```python
from build123d import *

# Parameters (mm, degrees)
SKETCH1_R                    = 1.6
BASE_DEPTH                   = 6
PTFE_CLAMP_3MM_OD_DEPTH      = 32.5
PTFE_CLAMP_1_6MM_OD_DEPTH    = 32.500000138
SKETCH3_R                    = 2.9
RUTHEX_M3_INSERT_HOLE_DEPTH  = 8.3
SIDE_PROFILE_DEPTH           = 4.4
ANGLE_CONSTRAINT_BACK_START  = -4
ANGLE_CONSTRAINT_BACK_DEPTH  = 8.4
ANGLE_CONSTRAINT_FRONT_START = -4
ANGLE_CONSTRAINT_FRONT_DEPTH = 8.4
FILLET4_R                    = 1
FILLET5_R                    = 2
FILLET4_OF_MIRROR4_R         = 1
FILLET5_OF_MIRROR4_R         = 2


with BuildPart() as part:
    # Sketch1 → base (new, symmetric)
    with BuildSketch(Plane(origin=(0, 0, 0), x_dir=(0, 0, -1), z_dir=(1, 0, 0))):
        with BuildLine():
            Line((7.5, 0), (-7.5, 0))
            Line((-7.5, 0), (-7.5, 22.5))
            ThreePointArc((-7.5, 22.5), (0, 30), (7.5, 22.5))
            Line((7.5, 22.5), (7.5, 0))
        make_face()
        with Locations((0, 22.5)):
            Circle(SKETCH1_R, mode=Mode.SUBTRACT)
    extrude(amount=BASE_DEPTH, both=True)

    # Sketch2 → PTFE_clamp_3mm_OD (cut, through all)
    with BuildSketch(Plane.XZ):
        with BuildLine():
            Line((0, -7.5), (1.202081528, -7.5))
            ThreePointArc((1.202081528, -7.5), (1.570595205, -5.647356637), (0, -4.597918472))
            Line((0, -4.597918472), (0, -7.5))
        make_face()
        with BuildLine():
            Line((-1.202081528, -7.5), (0, -7.5))
            Line((0, -7.5), (0, -4.597918472))
            ThreePointArc((0, -4.597918472), (-1.570595205, -5.647356637), (-1.202081528, -7.5))
        make_face()
        with BuildLine():
            Line((0, -7.5), (1.202081528, -7.5))
            ThreePointArc((1.202081528, -7.5), (1.570595205, -5.647356637), (0, -4.597918472))
            Line((0, -4.597918472), (0, -7.5))
        make_face()
        with BuildLine():
            Line((-1.202081528, -7.5), (0, -7.5))
            Line((0, -7.5), (0, -4.597918472))
            ThreePointArc((0, -4.597918472), (-1.570595205, -5.647356637), (-1.202081528, -7.5))
        make_face()
    extrude(amount=-PTFE_CLAMP_3MM_OD_DEPTH, mode=Mode.SUBTRACT)

    # Sketch2<3> → PTFE_clamp_1.6mm_OD (cut, through all)
    with BuildSketch(Plane.XZ):
        with BuildLine():
            ThreePointArc((-0.707106781, 7.5), (-0.923879533, 6.410209786), (0, 5.792893219))
            Line((0, 5.792893219), (0, 7.5))
            Line((0, 7.5), (-0.707106781, 7.5))
        make_face()
        with BuildLine():
            Line((0, 7.5), (0, 5.792893219))
            ThreePointArc((0, 5.792893219), (0.923879533, 6.410209786), (0.707106781, 7.5))
            Line((0.707106781, 7.5), (0, 7.5))
        make_face()
        with BuildLine():
            ThreePointArc((-0.707106781, 7.5), (-0.923879533, 6.410209786), (0, 5.792893219))
            Line((0, 5.792893219), (0, 7.5))
            Line((0, 7.5), (-0.707106781, 7.5))
        make_face()
        with BuildLine():
            Line((0, 7.5), (0, 5.792893219))
            ThreePointArc((0, 5.792893219), (0.923879533, 6.410209786), (0.707106781, 7.5))
            Line((0.707106781, 7.5), (0, 7.5))
        make_face()
    extrude(amount=-PTFE_CLAMP_1_6MM_OD_DEPTH, mode=Mode.SUBTRACT)

    # Sketch3 → ruthex_m3_insert_hole (cut)
    with BuildSketch(Plane.XZ):
        with Locations(Location((0, 0, 0), (0, 0, 270))):
            Circle(SKETCH3_R)
    extrude(amount=-RUTHEX_M3_INSERT_HOLE_DEPTH, mode=Mode.SUBTRACT)

    # Sketch4 → side_profile (add)
    with BuildSketch(Plane.ZY.offset(6)):
        Polygon((-8, 0), (7.5, 0), (7.5, 19.490381057), (3.077350269, 11.830127019), (-2.5, 11.830127019), (-8, 17.330127019), align=None)
    side_profile = extrude(amount=SIDE_PROFILE_DEPTH)

    # Sketch4<4> → angle_constraint_back (add)
    with BuildSketch(Plane.ZY.offset(6).offset(ANGLE_CONSTRAINT_BACK_START)):
        Polygon((-10.5, 0), (-8, 0), (-8, 17.330127019), (-8, 26.5), (-10.5, 26.5), align=None)
    angle_constraint_back = extrude(amount=ANGLE_CONSTRAINT_BACK_DEPTH)

    # Sketch4<6> → angle_constraint_front (add)
    with BuildSketch(Plane.ZY.offset(6).offset(ANGLE_CONSTRAINT_FRONT_START)):
        Polygon((7.5, 19.490381057), (7.5, 0), (10.5, 0), (10.5, 24.686533479), align=None)
    angle_constraint_front = extrude(amount=ANGLE_CONSTRAINT_FRONT_DEPTH)

    # Fillet4
    fillet4_edges = [part.edges().sort_by_distance(p)[0] for p in [
        (-6.2, 26.5, -8),
        (-6.2, 0, -10.5),
        (-6.2, 26.5, -10.5),
        (-6.2, 24.686533479, 10.5),
        (-6.2, 0, 10.5),
    ]]
    fillet(fillet4_edges, radius=FILLET4_R)

    # Fillet5
    # the kernel refuses this fillet: 2 mm, written as the material it adds along each edge
    with BuildSketch(Plane(origin=(-3.113248654, 11.830127019, 3.077350269), x_dir=(0, 0.8660254037844377, 0.5000000000000013), z_dir=(-1, 0, 0))) as fillet5_piece_1:
        with BuildLine():
            CenterArc((FILLET5_R * 0.57735026919, FILLET5_R), FILLET5_R, 210, 60)
            Line((-FILLET5_R * 0.288675134595, FILLET5_R * 0.5), (0, 0))
            Line((0, 0), (FILLET5_R * 0.57735026919, 0))
        make_face()
    extrude(amount=7.286751346)
    with BuildSketch(Plane(origin=(-3.928932188, 11.830127019, -2.5), x_dir=(0, 0.7071067811865489, -0.7071067811865462), z_dir=(-1, 0, 0))) as fillet5_piece_2:
        with BuildLine():
            CenterArc((FILLET5_R * 0.414213562373, -FILLET5_R), FILLET5_R, 90, 45)
            Line((-FILLET5_R * 0.292893218813, -FILLET5_R * 0.292893218813), (0, 0))
            Line((0, 0), (FILLET5_R * 0.414213562373, 0))
        make_face()
    extrude(amount=6.471067812)
    with BuildSketch(Plane(origin=(-6, 17.330127019, -8), x_dir=(0, 1, 0), z_dir=(-1, 0, 0))) as fillet5_piece_3:
        with BuildLine():
            CenterArc((FILLET5_R * 0.414213562373, -FILLET5_R), FILLET5_R, 90, 45)
            Line((-FILLET5_R * 0.292893218813, -FILLET5_R * 0.292893218813), (0, 0))
            Line((0, 0), (FILLET5_R * 0.414213562373, 0))
        make_face()
    extrude(amount=4.4)

    # Mirror4: side_profile, angle_constraint_back, angle_constraint_front across plane
    add(side_profile.mirror(Plane(origin=(0, 0, 0), x_dir=(0, 0, 1), z_dir=(1, 0, 0))))
    add(angle_constraint_back.mirror(Plane(origin=(0, 0, 0), x_dir=(0, 0, 1), z_dir=(1, 0, 0))))
    add(angle_constraint_front.mirror(Plane(origin=(0, 0, 0), x_dir=(0, 0, 1), z_dir=(1, 0, 0))))

    # Fillet4 of Mirror4
    fillet4_of_mirror4_edges = [part.edges().sort_by_distance(p)[0] for p in [
        (6.2, 26.5, -8),
        (6.2, 0, -10.5),
        (6.2, 26.5, -10.5),
        (6.2, 24.686533479, 10.5),
        (6.2, 0, 10.5),
    ]]
    fillet(fillet4_of_mirror4_edges, radius=FILLET4_OF_MIRROR4_R)

    # Fillet5 of Mirror4
    # the kernel refuses this fillet: 2 mm, written as the material it adds along each edge
    with BuildSketch(Plane(origin=(3.113248654, 11.830127019, 3.077350269), x_dir=(0, 0.8660254037844386, 0.5000000000000002), z_dir=(1, 0, 0))) as fillet5_of_mirror4_piece_1:
        with BuildLine():
            CenterArc((FILLET5_OF_MIRROR4_R * 0.57735026919, -FILLET5_OF_MIRROR4_R), FILLET5_OF_MIRROR4_R, 90, 60)
            Line((-FILLET5_OF_MIRROR4_R * 0.288675134595, -FILLET5_OF_MIRROR4_R * 0.5), (0, 0))
            Line((0, 0), (FILLET5_OF_MIRROR4_R * 0.57735026919, 0))
        make_face()
    extrude(amount=7.286751346)
    with BuildSketch(Plane(origin=(3.928932188, 11.830127019, -2.5), x_dir=(0, 0, 1), z_dir=(1, 0, 0))) as fillet5_of_mirror4_piece_2:
        with BuildLine():
            CenterArc((FILLET5_OF_MIRROR4_R * 0.414213562373, -FILLET5_OF_MIRROR4_R), FILLET5_OF_MIRROR4_R, 90, 45)
            Line((-FILLET5_OF_MIRROR4_R * 0.292893218813, -FILLET5_OF_MIRROR4_R * 0.292893218813), (0, 0))
            Line((0, 0), (FILLET5_OF_MIRROR4_R * 0.414213562373, 0))
        make_face()
    extrude(amount=6.471067812)
    with BuildSketch(Plane(origin=(6, 17.330127019, -8), x_dir=(0, 1, 0), z_dir=(1, 0, 0))) as fillet5_of_mirror4_piece_3:
        with BuildLine():
            CenterArc((FILLET5_OF_MIRROR4_R * 0.414213562373, FILLET5_OF_MIRROR4_R), FILLET5_OF_MIRROR4_R, 225, 45)
            Line((-FILLET5_OF_MIRROR4_R * 0.292893218813, FILLET5_OF_MIRROR4_R * 0.292893218813), (0, 0))
            Line((0, 0), (FILLET5_OF_MIRROR4_R * 0.414213562373, 0))
        make_face()
    extrude(amount=4.4)


solid = part.part
```
The listing builds one solid part. Answer for the finished solid, in the listing's coordinates (mm). A direction names the side the tool comes from. Round coordinates to 2 decimals unless told otherwise and drop trailing zeros. Write each loop counter-clockwise with the first axis right and the second up, starting at its lowest first coordinate (ties: lowest second). Pieces come first, ordered by that corner, then holes. Notation, with made-up numbers: (22.25, 83.5) -> (54.25, 83.5) arc R34 ccw to (54.25, 113.5) -> close; hole circle Ø10 at (32.5, -3.5). An arc over 180 degrees is marked (long way). Answer as a JSON object with one key per item and string values. Group by question number.
Q1. Each of these flat-tipped pins is pushed along its axis until it touches: pin 1 Ø1.8 at (x, z) = (9, 0.5) entering from +Y; pin 2 Ø4.5 at (x, z) = (0, 0) entering from -Y; pin 3 Ø1.5 at (x, z) = (-1, 2.5) entering from +Y; pin 4 Ø5 at (x, z) = (1, -2) entering from +Y. Where does it stop, or does it pass through?
Q2. Section C-C (x = -7.25) is taken. Write down the section's boundary in (y, z), plus the area to 3 significant figures.
Q3. Straight lines are drawn through the part: line 1 along Y through (x, z) = (-0.75, 0); line 2 along X through (y, z) = (5, 0); line 3 along Z through (x, y) = (-4.25, 12). For each, find the intervals that lie inside material, in ascending order.
Q4. Section D-D (y = 20.5) is taken. Write down the section's boundary in (x, z), plus the area to 3 significant figures.
Q5. Determine the mould class of faces 4 (the face through (-1.6, 13.7, 7.5)), 5 (the face through (5, 15, -8)), 6 (the face through (6, 11, 10.5)) for opening direction X: pulls with the +X half, pulls with the -X half, needs draft (parallel to the pull), parting line crosses it, or undercut.
Q6. Section A-A (z = 0) is taken. Write down the section's boundary in (x, y), plus the area to 3 significant figures.
Q7. Section B-B (y = 3) is taken. Write down the section's boundary in (x, z).
Q8. Which of the six approach directions +Z, -Z, +X, -X, +Y, -Y give full straight-line access (tool end or side, diameter ignored) to faces 1 (the face through (2, 11, 9)), 2 (the face through (2, 13, -9)), 3 (the face through (-8.17, 12.09, 2.91))?
Check values:
{
 "1": {"pin 1": "y = 11.83", "pin 2": "y = 8.3", "pin 3": "y = 29.79", "pin 4": "y = 30"},
 "2": {"outline": "(0, -9.5) arc R1 ccw to (1, -10.5) -> (25.5, -10.5) arc R1 ccw to (26.5, -9.5) -> (26.5, -9) arc R1 ccw to (25.5, -8) -> (18.16, -8) arc R2 cw to (16.74, -7.41) -> (12.42, -3.09) arc R2 cw to (11.83, -1.67) -> (11.83, 1.92) arc R2 cw to (12.83, 3.65) -> (21.45, 8.63) arc R1 ccw to (20.95, 10.5) -> (1, 10.5) arc R1 ccw to (0, 9.5) -> close", "area": "345 mm^2"},
 "3": {"line 1": "8.3 to 20.9, 24.1 to 30", "line 2": "-10.4 to -2.9, 2.9 to 10.4", "line 3": "-10.5 to -8, -7.5 to 10.5"},
 "4": {"outline": "(-10.4, -10.5) -> (-2, -10.5) -> (-2, -8) -> (-10.4, -8) -> close; (-10.4, 8.08) -> (-2, 8.08) -> (-2, 10.5) -> (-10.4, 10.5) -> close; (-6, -7.5) -> (-1.2, -7.5) arc R1.7 cw (long way) to (1.2, -7.5) -> (6, -7.5) -> (6, 7.5) -> (0.71, 7.5) arc R1 cw (long way) to (-0.71, 7.5) -> (-6, 7.5) -> close; (2, -10.5) -> (10.4, -10.5) -> (10.4, -8) -> (2, -8) -> close; (2, 8.08) -> (10.4, 8.08) -> (10.4, 10.5) -> (2, 10.5) -> close", "area": "251 mm^2"},
 "5": {"face 4": "undercut", "face 5": "undercut", "face 6": "needs draft"},
 "6": {"outline": "(-10.4, 0) -> (-2.9, 0) -> (-2.9, 8.3) -> (2.9, 8.3) -> (2.9, 0) -> (10.4, 0) -> (10.4, 11.83) -> (6, 11.83) -> (6, 20.9) -> (-6, 20.9) -> (-6, 11.83) -> (-10.4, 11.83) -> close; (-6, 24.1) -> (6, 24.1) -> (6, 30) -> (-6, 30) -> close", "area": "378 mm^2"},
 "7": {"outline": "(-10.4, -10.5) -> (-2, -10.5) -> (-2, -8) -> (-6, -8) -> (-6, -7.5) -> (-1.2, -7.5) arc R1.7 cw (long way) to (1.2, -7.5) -> (6, -7.5) -> (6, -8) -> (2, -8) -> (2, -10.5) -> (10.4, -10.5) -> (10.4, 10.5) -> (2, 10.5) -> (2, 7.5) -> (0.71, 7.5) arc R1 cw (long way) to (-0.71, 7.5) -> (-2, 7.5) -> (-2, 10.5) -> (-10.4, 10.5) -> close; hole circle Ø5.8 at (0, 0)"},
 "8": {"face 1": "+Z, +Y, -Y", "face 2": "-Z, +Y, -Y", "face 3": "-X, +Y"}
}
